```python
from build123d import *

# Parameters (mm, degrees)
EXTRUDE_1_DEPTH             = 26
CUT_EXTRUDE_3_DEPTH         = 8
PATTERN_LINEAR_3_COUNT      = 3
PATTERN_LINEAR_3_PITCH      = 50
PATTERN_LINEAR_3_COUNT_DIR2 = 3
PATTERN_LINEAR_3_PITCH_DIR2 = 50
CHAMFER_3_SIZE              = 1
SKETCH_5_R                  = 4


with BuildPart() as part:
    # 草图1 → 凸台-拉伸1 (new body)
    with BuildSketch(Plane(origin=(0, 0, 0), x_dir=(1, 0, 0), z_dir=(0, 1, 0))):
        with BuildLine():
            Line((-90, 250), (90, 250))
            ThreePointArc((90, 250), (97.071067812, 247.071067812), (100, 240))
            Line((100, 240), (100, 20))
            ThreePointArc((100, 20), (102.928932188, 12.928932188), (110, 10))
            Line((110, 10), (127, 10))
            ThreePointArc((127, 10), (129.121320344, 9.121320344), (130, 7))
            Line((130, 7), (130, 0))
            Line((130, 0), (-130, 0))
            Line((-130, 0), (-130, 7))
            ThreePointArc((-130, 7), (-129.121320344, 9.121320344), (-127, 10))
            Line((-127, 10), (-110, 10))
            ThreePointArc((-110, 10), (-102.928932188, 12.928932188), (-100, 20))
            Line((-100, 20), (-100, 240))
            ThreePointArc((-100, 240), (-97.071067812, 247.071067812), (-90, 250))
        make_face()
    extrude(amount=EXTRUDE_1_DEPTH)

    # 草图3 → 切除-拉伸3 (cut)
    with BuildSketch(Plane(origin=(0, 26, 0), x_dir=(1, 0, 0), z_dir=(0, 1, 0))):
        with BuildLine():
            Line((-67, 230), (-33, 230))
            ThreePointArc((-33, 230), (-30.878679656, 229.121320344), (-30, 227))
            Line((-30, 227), (-30, 193))
            ThreePointArc((-30, 193), (-30.878679656, 190.878679656), (-33, 190))
            Line((-33, 190), (-67, 190))
            ThreePointArc((-67, 190), (-69.121320344, 190.878679656), (-70, 193))
            Line((-70, 193), (-70, 227))
            ThreePointArc((-70, 227), (-69.121320344, 229.121320344), (-67, 230))
        make_face()
    cut_extrude_3 = extrude(amount=-CUT_EXTRUDE_3_DEPTH, mode=Mode.SUBTRACT)

    # 阵列(线性)3: Cut-Extrude 3 3 × 3
    with Locations(*[(i * PATTERN_LINEAR_3_PITCH, 0, j * PATTERN_LINEAR_3_PITCH_DIR2) for i in range(PATTERN_LINEAR_3_COUNT) for j in range(PATTERN_LINEAR_3_COUNT_DIR2) if (i, j) != (0, 0)]):
        add(cut_extrude_3, mode=Mode.SUBTRACT)

    # 倒角3
    chamfer_3_edges = [part.edges().sort_by_distance(p)[0] for p in [
        (-30.878679656, 26, -140.878679656),
        (-50, 26, -140),
        (-69.121320344, 26, -140.878679656),
        (-70, 26, -160),
        (-69.121320344, 26, -179.121320344),
        (-50, 26, -180),
        (-30.878679656, 26, -179.121320344),
        (-30, 26, -160),
        (19.121320344, 26, -140.878679656),
        (0, 26, -140),
        (-19.121320344, 26, -140.878679656),
        (-20, 26, -160),
        (-19.121320344, 26, -179.121320344),
        (0, 26, -180),
        (19.121320344, 26, -179.121320344),
        (20, 26, -160),
        (97.071067812, 26, -247.071067812),
        (69.121320344, 26, -140.878679656),
        (50, 26, -140),
        (30.878679656, 26, -140.878679656),
        (30, 26, -160),
        (30.878679656, 26, -179.121320344),
        (50, 26, -180),
        (69.121320344, 26, -179.121320344),
        (70, 26, -160),
        (-30.878679656, 26, -90.878679656),
        (-50, 26, -90),
        (-69.121320344, 26, -90.878679656),
        (-70, 26, -110),
        (-69.121320344, 26, -129.121320344),
        (-50, 26, -130),
        (-30.878679656, 26, -129.121320344),
        (-30, 26, -110),
        (0, 26, -250),
        (19.121320344, 26, -90.878679656),
        (0, 26, -90),
        (-19.121320344, 26, -90.878679656),
        (-20, 26, -110),
        (-19.121320344, 26, -129.121320344),
        (0, 26, -130),
        (19.121320344, 26, -129.121320344),
        (20, 26, -110),
        (69.121320344, 26, -90.878679656),
        (50, 26, -90),
        (30.878679656, 26, -90.878679656),
        (30, 26, -110),
        (30.878679656, 26, -129.121320344),
        (50, 26, -130),
        (69.121320344, 26, -129.121320344),
        (70, 26, -110),
        (-97.071067812, 26, -247.071067812),
        (-100, 26, -130),
        (-102.928932188, 26, -12.928932188),
        (-118.5, 26, -10),
        (-129.121320344, 26, -9.121320344),
        (-130, 26, -3.5),
        (0, 26, 0),
        (-30.878679656, 26, -190.878679656),
        (-30, 26, -210),
        (-30.878679656, 26, -229.121320344),
        (130, 26, -3.5),
        (-50, 26, -230),
        (-69.121320344, 26, -229.121320344),
        (-70, 26, -210),
        (-69.121320344, 26, -190.878679656),
        (102.928932188, 26, -12.928932188),
        (-50, 26, -190),
        (129.121320344, 26, -9.121320344),
        (118.5, 26, -10),
        (19.121320344, 26, -190.878679656),
        (20, 26, -210),
        (19.121320344, 26, -229.121320344),
        (0, 26, -230),
        (-19.121320344, 26, -229.121320344),
        (-20, 26, -210),
        (-19.121320344, 26, -190.878679656),
        (0, 26, -190),
        (69.121320344, 26, -190.878679656),
        (50, 26, -190),
        (30.878679656, 26, -190.878679656),
        (30, 26, -210),
        (30.878679656, 26, -229.121320344),
        (50, 26, -230),
        (69.121320344, 26, -229.121320344),
        (70, 26, -210),
        (100, 26, -130),
    ]]
    chamfer(chamfer_3_edges, length=CHAMFER_3_SIZE)

    # 扫描1: sweep along a path in 草图4
    with BuildLine(Plane(origin=(0, 12, 0), x_dir=(-1, 0, 0), z_dir=(0, -1, 0))) as sweep_1_path:
        Line((-40, 0), (-40, -4))
        ThreePointArc((-40, -4), (-36.485281374, -12.485281374), (-28, -16))
        Line((-28, -16), (28, -16))
        ThreePointArc((28, -16), (36.485281374, -12.485281374), (40, -4))
        Line((40, -4), (40, 0))
    # 草图5 → 扫描1 (sweep)
    with BuildSketch(Plane.XY):
        with Locations((-40, 12)):
            Circle(SKETCH_5_R)
    sweep(path=sweep_1_path.line)


solid = part.part
```
Could you check a few things on this model? Use its own coordinates, in mm. A direction names the side the tool comes from. Round coordinates to 2 decimals unless told otherwise and drop trailing zeros. Loops run counter-clockwise (first coordinate to the right, second up) from the corner with the lowest first, then second, coordinate; pieces in that order, holes last. Notation, with made-up numbers: M 7,-7 L 15,-7 A12 cw 15,14 Z; hole C 52,24.25 d6. An arc over 180 degrees is marked long. Write item = value, one per line.
1. Which directions (+Z, -Z, +X, -X, +Y, -Y) give clear straight access to the entire face, cutting with the end or side of a thin tool? Please do faces 1 (the face through (-30, 22, -110)), 2 (the face through (-130, 12, -3)).
Results below:
face_1 = +Y
face_2 = +Z, -Z, -X, +Y, -Y
2. I want a section at A-A, the plane y = 12. Write out the boundary of the cut face in (x, z), and give its area (3 significant figures).
Results below:
outline = M -130,-7 A3 ccw -127,-10 L -110,-10 A10 cw -100,-20 L -100,-240 A10 ccw -90,-250 L 90,-250 A10 ccw 100,-240 L 100,-20 A10 cw 110,-10 L 127,-10 A3 ccw 130,-7 L 130,0 L 44,0 L 44,4 A16 ccw 28,20 L -28,20 A16 ccw -44,4 L -44,0 L -130,0 Z; hole M -36,0 L 36,0 L 36,4 A8 ccw 28,12 L -28,12 A8 ccw -36,4 Z
area = 51,400 mm²
3. I want a section at B-B, the plane z = -166. Write out the boundary of the cut face in (x, y).
Results below:
outline = M -100,0 L 100,0 L 100,25 L 99,26 L 71,26 L 70,25 L 70,18 L 30,18 L 30,25 L 29,26 L 21,26 L 20,25 L 20,18 L -20,18 L -20,25 L -21,26 L -29,26 L -30,25 L -30,18 L -70,18 L -70,25 L -71,26 L -99,26 L -100,25 Z
4. I need wall thicknesses on probe 1 along X at (y, z) = (24.75, -124); probe 2 along Z at (x, y) = (35.5, 20.5); probe 3 along Y at (x, z) = (-11.5, -176.5). Which ranges of each line are inside material? Lowest first, please.
Results below:
probe_1 = -100 to -70, -30 to -20, 20 to 30, 70 to 100
probe_2 = -250 to -230, -190 to -180, -140 to -130, -90 to 0
probe_3 = 0 to 18
5. Will these pins go through, and if not, where does the flat tip stop? P1, Ø3.5, axis at x = 48, y = 23, coming from the +Z side; P2, Ø2, axis at y = 21.5, z = -157, coming from the -X side; P3, Ø7.5, axis at y = 20, z = -164, coming from the +X side.
Results below:
P1 = 0
P2 = -100
P3 = 100
6. Thinking about a two-plate mould opening in Z: for faces 3 (the face through (-30, 22, -160)), 4 (the face through (102.85, 12.32, -13.01)), 5 (the face through (-100, 12, -128)), which applies, +Z half, -Z half, draft (parallel to the pull), parting line (faces both ways), or undercut?
Results below:
face_3 = undercut
face_4 = -Z half
face_5 = draft
7. I want a section at C-C, the plane z = -63.5. Write out the boundary of the cut face in (x, y), and give its area (3 significant figures).
Results below:
outline = M -100,0 L 100,0 L 100,25 L 99,26 L -99,26 L -100,25 Z
area = 5,200 mm²
